Study the drawing (mm; zero at the part's minimum x, y, z) and answer. Coordinates: 2 decimals unless noted, no trailing zeros. Write each loop counter-clockwise with the first axis right and the second up, starting at its lowest first coordinate (ties: lowest second). Pieces come first, ordered by that corner, then holes. Notation, with made-up numbers: (24.5, 43) -> (45.5, 43) arc R27 cw to (45.5, 61) -> close; hole circle Ø9 at (-11.5, 11). An arc over 180 degrees is marked (long way). Answer in a Markdown table with one row per item. Add a question column.
Item 1: Section B-B on x = 101.6 is taken. Write down the section's boundary in (y, z) (3 decimals), then the cut area to 3 significant figures.
Item 2: Given pin 1 Ø4 at (x, y) = (141.097, 101.6) entering from -Z, flat-ended and moving along its own axis, determine where the tip first touches the part or whether it passes through.
Item 3: Straight lines are drawn through the part: line 1 (X direction, y = 102, z = 10.5); line 2 (Y direction, x = 101.6, z = 7.5) (3 decimals); line 3 (X direction, y = 95, z = 1.25). For each, find the intervals that lie inside material, in ascending order. Write a range as from..to.
Item 4: Section A-A on y = 101.6 is taken. Write down the section's boundary in (x, z) (3 decimals), then the cut area to 3 significant figures.
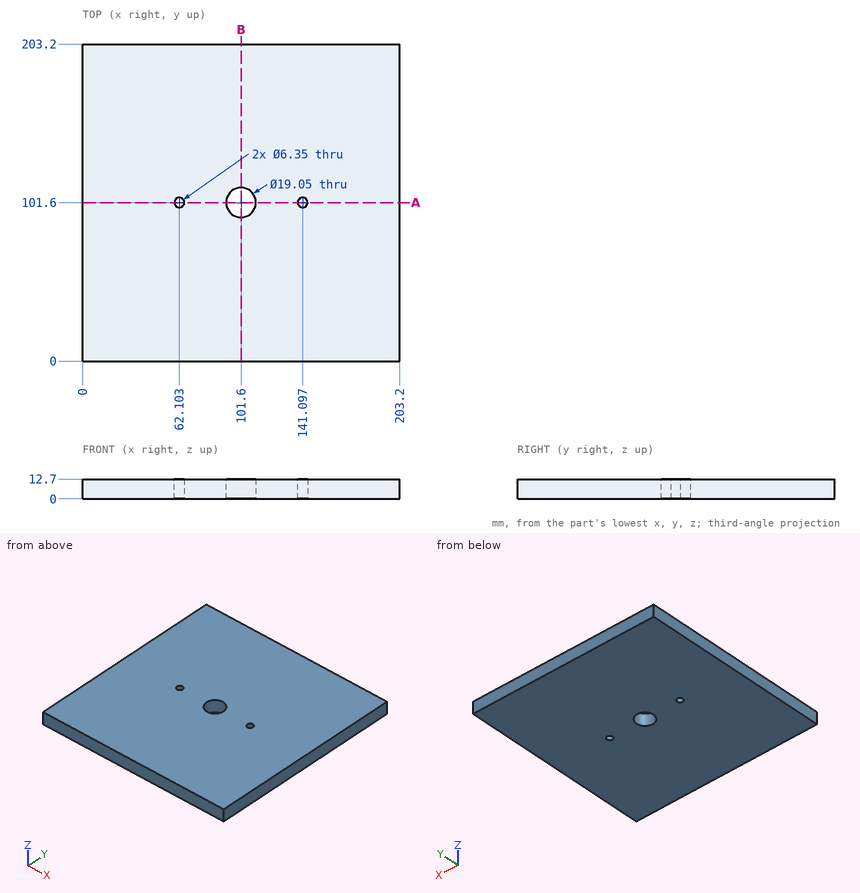
Results below:
| question | item | result |
|---|---|---|
| 1 | outline | (0, 0) -> (92.075, 0) -> (92.075, 12.7) -> (0, 12.7) -> close; (111.125, 0) -> (203.2, 0) -> (203.2, 12.7) -> (111.125, 12.7) -> close |
| 1 | area | 2,340 mm2 |
| 2 | pin 1 | passes through |
| 3 | line 1 | x = 0..58.95, 65.25..92.08, 111.12..137.95, 144.25..203.2 |
| 3 | line 2 | y = 0..92.075, 111.125..203.2 |
| 3 | line 3 | x = 0..94.73, 108.47..203.2 |
| 4 | outline | (0, 0) -> (58.928, 0) -> (58.928, 12.7) -> (0, 12.7) -> close; (65.278, 0) -> (92.075, 0) -> (92.075, 12.7) -> (65.278, 12.7) -> close; (111.125, 0) -> (137.922, 0) -> (137.922, 12.7) -> (111.125, 12.7) -> close; (144.272, 0) -> (203.2, 0) -> (203.2, 12.7) -> (144.272, 12.7) -> close |
| 4 | area | 2,180 mm2 |
